Autodesk Inventor part; units mm, degrees
ref_plane "YZ Plane" through (0, 0, 0) normal (1, 0, 0) x (0, 1, 0)
ref_plane "XZ Plane" through (0, 0, 0) normal (0, 1, 0) x (-1, 0, 0)
ref_plane "XY Plane" through (0, 0, 0) normal (0, 0, 1) x (1, 0, 0)
sketch "Skizze1" plane through (0, 0, 0) normal (0, 1, 0) x (-1, 0, 0)
  line L0 (0, 0) -> (12, 0)
  line L1 (12, 0) -> (12, -16)
  line L2 (12, -16) -> (0, -16)
  line L3 (0, -16) -> (0, 0)
  line L4 (17, 5) -> (17, -21)
  line L5 (-5, -21) -> (-5, 5)
  line L6 (-1, 1) -> (13, 1)
  line L7 (13, 1) -> (13, -17)
  line L8 (13, -17) -> (-1, -17)
  line L9 (-1, -17) -> (-1, 1)
  line L10 (1.75, -1.75) -> (10.25, -1.75)
  line L11 (10.25, -1.75) -> (10.25, -14.25)
  line L12 (10.25, -14.25) -> (1.75, -14.25)
  line L13 (1.75, -14.25) -> (1.75, -1.75)
  line L14 (0.75, -0.75) -> (11.25, -0.75)
  line L15 (11.25, -0.75) -> (11.25, -15.25)
  line L16 (11.25, -15.25) -> (0.75, -15.25)
  line L17 (0.75, -15.25) -> (0.75, -0.75)
  line L18 (15.25, 5.25) -> (-3.25, 5.25)
  line L19 (-3.25, 5.25) -> (-3.25, -21.25)
  line L20 (-3.25, -21.25) -> (15.25, -21.25)
  line L21 (15.25, -21.25) -> (15.25, 5.25)
  line L22 (16.25, 6.25) -> (-4.25, 6.25)
  line L23 (-4.25, 6.25) -> (-4.25, -22.25)
  line L24 (-4.25, -22.25) -> (16.25, -22.25)
  line L25 (16.25, -22.25) -> (16.25, 6.25)
  point P0 (6, 0)
  point P1 (6, 5)
  point P2 (6, -16)
  point P3 (12, -8)
  point P4 (6, -1.75)
  point P5 (6, -14.25)
  point P6 (10.25, -8)
  point P7 (1.75, -8)
  point P8 (6, -21.25)
  dimension "d0" = 16
  dimension "d1" = 12
  dimension "d2" = 5
  dimension "d3" = 5
  dimension "d56" = 1
  dimension "d57" = 1
  dimension "d58" = 1
  dimension "d60" = 1.75
  dimension "d61" = 1.75
  dimension "d63" = 8.5
  dimension "d64" = 1
  dimension "d65" = 1
  dimension "d67" = 1
  dimension "d69" = 12.5
  dimension "d70" = 1
  dimension "d71" = 1.75
  dimension "d72" = 1.75
  dimension "d74" = 7
  dimension "d76" = 7
  dimension "d77" = 5
  dimension "d78" = 5
  dimension "d80" = 1
  dimension "d81" = 1
  dimension "d82" = 1
  dimension "d83" = 1
ref_plane "Arbeitsebene1" through (0, 0, 0) normal (0, -1, 0) x (1, 0, 0)
sketch "Skizze2" plane through (0, 0, 0) normal (0, -1, 0) x (1, 0, 0)
  line L0 (21, 19) -> (-33, 19)
  line L1 (-33, 19) -> (-33, -35)
  line L2 (-33, -35) -> (21, -35)
  line L3 (21, -35) -> (21, 19)
  line L4 (-17, -21) -> (-17, 5)
  line L5 (5, -21) -> (-17, -21)
  line L6 (5, 5) -> (5, -21)
  line L7 (-17, 5) -> (5, 5)
  point P0 (0, 0)
  dimension "d11" = 16
  dimension "d12" = 14
  dimension "d13" = 16
  dimension "d14" = 14
  dimension "d35" = 54
  dimension "d36" = 54
extrude "Extrusion2" add sketch "Skizze2" along normal blind 5 contours L3 L2 L1 L0 | L4 L7 L6 L5
ref_plane "Arbeitsebene2" through (0, 0, 0) normal (0, 1, 0) x (1, 0, 0)
sketch "Skizze4" plane through (0, 0, 0) normal (0, 1, 0) x (1, 0, 0)
  line L0 (21, 35) -> (21, -19)
  line L1 (-33, 35) -> (21, 35)
  line L2 (21, -19) -> (-33, -19)
  line L3 (-33, -19) -> (-33, 35)
  point P0 (0, 0)
  point P1 (14, 28)
  point P2 (14, -12)
  point P3 (-26, -12)
  point P4 (-26, 28)
  dimension "d44" = 7
  dimension "d45" = 7
  dimension "d46" = 7
  dimension "d47" = 7
  dimension "d48" = 7
  dimension "d49" = 7
  dimension "d50" = 7
  dimension "d51" = 7
  dimension "d52" = 40
  dimension "d53" = 40
  dimension "d54" = 40
  dimension "d55" = 40
hole "Bohrung1" at (14, 0, -28) at (14, 0, 12) at (-26, 0, 12) at (-26, 0, -28) direction (0, -1, 0) diameter 8.5 depth 5
extrude "Extrusion4" add sketch "Skizze1" along normal blind 4 contours L25 L24 L23 L22
properties part number "Magazin_1_3D-Druck"
Source: CAD feature listing. Evaluate the final solid. Frame: model axes, mm. A direction names the side the tool comes from. Coordinates: 2 decimals unless noted, no trailing zeros. Write each loop counter-clockwise with the first axis right and the second up, starting at its lowest first coordinate (ties: lowest second). Pieces come first, ordered by that corner, then holes. Notation, with made-up numbers: M 16.25,-5 L 23.25,-5 A31 cw 23.25,25 Z; hole C 16,72 d1. An arc over 180 degrees is marked long. Use a Markdown table: item, result.
1) Section B-B, the plane z = -28. Output: boundary loops of the cut face in (x, y), then the cut area to 3 significant figures.
Conclusion:
| item | result |
|---|---|
| outline | M -33,-5 L -30.25,-5 L -30.25,0 L -33,0 Z; M -21.75,-5 L 9.75,-5 L 9.75,0 L -21.75,0 Z; M 18.25,-5 L 21,-5 L 21,0 L 18.25,0 Z |
| area | 185 mm^2 |
2) Section A-A, the plane x = 14. Output: boundary loops of the cut face in (y, z), then the cut area to 3 significant figures.
Conclusion:
| item | result |
|---|---|
| outline | M -5,-35 L 0,-35 L 0,-32.25 L -5,-32.25 Z; M -5,-23.75 L 0,-23.75 L 0,7.75 L -5,7.75 Z; M -5,16.25 L 0,16.25 L 0,19 L -5,19 Z |
| area | 185 mm^2 |
3) Reachability of faces 1 (the flat face through (3.25, 2, -8)), 2 (the flat face through (4.25, 2, -8)), 3 (the flat face through (-16.25, 2, -8)) from +Z, -Z, +X, -X, +Y, -Y: full face, straight path, thin tool, end or side. Return the list, or none.
Conclusion:
| item | result |
|---|---|
| face 1 | +Y |
| face 2 | +Z, -Z, +X, +Y |
| face 3 | +Z, -Z, -X, +Y |
4) Section D-D, the plane y = -4. Output: boundary loops of the cut face in (x, z), then the cut area to 3 significant figures.
Conclusion:
| item | result |
|---|---|
| outline | M -33,-35 L 21,-35 L 21,19 L -33,19 Z; hole C -26,-28 d8.5; hole C -26,12 d8.5; hole C 14,-28 d8.5; hole C 14,12 d8.5 |
| area | 2,690 mm^2 |
5) Section C-C, the plane y = 2. Output: boundary loops of the cut face in (x, z).
Conclusion:
| item | result |
|---|---|
| outline | M -16.25,-22.25 L 4.25,-22.25 L 4.25,6.25 L -16.25,6.25 Z; hole M -15.25,-21.25 L 3.25,-21.25 L 3.25,5.25 L -15.25,5.25 Z |
6) Ray query, L1, parallel to Z at x = -26, y = -1.5; L2, parallel to X at y = -1.9, z = -28; L3, parallel to X at y = 3.75, z = 0. Return the intervals inside material, ascending.
Conclusion:
| item | result |
|---|---|
| L1 | z = -35 to -32.25, -23.75 to 7.75, 16.25 to 19 |
| L2 | x = -33 to -30.25, -21.75 to 9.75, 18.25 to 21 |
| L3 | x = -16.25 to -15.25, 3.25 to 4.25 |
7) First-contact query: pin 1 Ø20.5 at (x, z) = (-8.5, -4.5) entering from +Y; pin 2 Ø11 at (x, z) = (14, 12) entering from +Y; pin 3 Ø2 at (y, z) = (3, -3.5) entering from -X; pin 4 Ø1.2 at (x, y) = (-3, 3) entering from +Z. Flat tips, straight axial feed; report the tip coordinate or a pass-through.
Conclusion:
| item | result |
|---|---|
| pin 1 | stops at y = 4 |
| pin 2 | stops at y = 0 |
| pin 3 | stops at x = -16.25 |
| pin 4 | stops at z = 6.25 |
8) Mould query, pull axis Z, two halves, no side actions, for faces 4 (the flat face through (4, 4, -8)), 5 (the cylindrical face through (-30.214, -2.535, 11.447)), 6 (the flat face through (-6, 2, 6.25)). Classes: pulls with the +Z half, pulls with the -Z half, needs draft (parallel to the pull), parting line crosses it, or undercut.
Conclusion:
| item | result |
|---|---|
| face 4 | needs draft |
| face 5 | undercut |
| face 6 | pulls with the +Z half |
